Input: part model. Units: mm. Frame: model coordinates. A direction names the side the tool comes from. Coordinates: 2 decimals unless noted, no trailing zeros. Write each loop counter-clockwise with the first axis right and the second up, starting at its lowest first coordinate (ties: lowest second). Pieces come first, ordered by that corner, then holes. Notation, with made-up numbers: M 10,39.5 L 53,39.5 A12 ccw 53,58.5 Z; hole C 33.5,3 d10. An arc over 180 degrees is marked long. Use one line per item in the form item = value.
from build123d import *

# Parameters (mm, degrees)
F3_DEPTH = 25.4
F4_R     = 9.525
F5_DEPTH = 20.828
F6_SIZE  = 1.5875


with BuildPart() as f1:
    # F0 (on Front) → F1 (revolve)
    with BuildSketch(Plane.XZ):
        with BuildLine():
            Line((-98.425, 19.05), (-98.425, 0))
            Line((-98.425, 0), (98.425, 0))
            ThreePointArc((98.425, 0), (92.845384, 13.470384), (79.375, 19.05))
            Line((79.375, 19.05), (-98.425, 19.05))
        make_face()
    revolve(axis=Axis((0, 0, 0), (1, 0, 0)))

    # F2 (on Top) → F3 (cut)
    with BuildSketch(Plane.XY):
        with BuildLine():
            Line((79.375, 19.05), (58.547, 19.05))
            Line((58.547, 19.05), (58.547, -19.05))
            Line((58.547, -19.05), (79.375, -19.05))
            ThreePointArc((79.375, -19.05), (98.425, 0), (79.375, 19.05))
        make_face()
    extrude(amount=F3_DEPTH, mode=Mode.SUBTRACT)

    # F4 (on face) → F5 (join)
    with BuildSketch(Plane.XY):
        with Locations((79.375, 0)):
            Circle(F4_R)
    extrude(amount=F5_DEPTH)

    # F6
    f6_edges = [f1.edges().sort_by_distance(p)[0] for p in [
        (69.85, 0, 20.828),
    ]]
    chamfer(f6_edges, length=F6_SIZE)


solid = f1.part
(1) Line query: probe 1 along Y at (x, z) = (-60, -16.5); probe 2 along X at (y, z) = (-18, 1) (3 decimals); probe 3 along X at (y, z) = (-5.5, 3.5) (3 decimals). Output: solid intervals per line, ascending.
Computed:
probe_1 = -9.52 to 9.52
probe_2 = -98.425 to 58.547
probe_3 = -98.425 to 58.547, 71.598 to 87.152
(2) Section query B-B on x = 3. Return the cut outline in (y, z).
Computed:
outline = C 0,0 d38.1
(3) First-contact query: pin 1 Ø2 at (x, y) = (58, 3.5) entering from -Z; pin 2 Ø4 at (x, z) = (23, -9) entering from -Y; pin 3 Ø6 at (x, z) = (3.5, -10) entering from +Y. Flat tips, straight axial feed; report the tip coordinate or a pass-through.
Computed:
pin_1 = -18.89
pin_2 = -17.72
pin_3 = 17.72
(4) Section query D-D on x = 68. Return the cut outline in (y, z).
Computed:
outline = M -19.05,0 A19.05 ccw 19.05,0 Z
(5) Pull-direction query (X, two-part tool) for faces 1 (the cylindrical face through (-10.77, -0.84, -19.03)), 2 (the flat face through (58.547, 0, 7)), 3 (the cylindrical face through (69.86, 0.42, 9.49)), 4 (the flat face through (-98.425, 0, 0)); classes: pulls with the +X half, pulls with the -X half, needs draft (parallel to the pull), parting line crosses it, or undercut.
Computed:
face_1 = needs draft
face_2 = undercut
face_3 = undercut
face_4 = pulls with the -X half
(6) Section query C-C on z = 5. Return the cut outline in (x, y) (3 decimals).
Computed:
outline = M -98.425,-18.382 L 58.547,-18.382 L 58.547,18.382 L -98.425,18.382 Z; C 79.375,0 d19.05
(7) Set-up query: faces 5 (the flat face through (79, 0, 20.828)), 6 (the flat face through (69, 0, 0)). Return all of +Z, -Z, +X, -X, +Y, -Y with unobstructed straight access to the full face (end or side cutting, diameter ignored); none if empty.
Computed:
face_5 = +Z, +X, -X, +Y, -Y
face_6 = +Z
(8) Section query A-A on z = 16.5. Return the cut outline in (x, y) (3 decimals), plus the area to 3 significant figures.
Computed:
outline = M -98.425,-9.521 L 58.547,-9.521 L 58.547,9.521 L -98.425,9.521 Z; C 79.375,0 d19.05
area = 3,270 mm^2
